Model file for the job. Use its own axes, mm. Round coordinates to 2 decimals unless told otherwise and drop trailing zeros. Loops run counter-clockwise (first coordinate to the right, second up) from the corner with the lowest first, then second, coordinate; pieces in that order, holes last. Notation, with made-up numbers: (51.5, 76.25) -> (58.5, 76.25) arc R13 ccw to (58.5, 96.25) -> close; hole circle Ø2 at (22.25, 82). An arc over 180 degrees is marked (long way). Use a Markdown table: item, result. Add a question column.
```python
from build123d import *

# Parameters (mm, degrees)
SKIZZE1_R                       = 2.25
AUFSATZ_LINEAR_AUSTRAGEN1_DEPTH = 20
SKIZZE2_R                       = 3
AUFSATZ_LINEAR_AUSTRAGEN2_DEPTH = 1
AUFSATZ_LINEAR_START            = 1
SKIZZE3_R                       = 3
AUFSATZ_LINEAR_AUSTRAGEN3_DEPTH = 1


with BuildPart() as part:
    # Skizze1 → Aufsatz-Linear austragen1 (new body)
    with BuildSketch(Plane.XY):
        with Locations((-14.9, 25)):
            Circle(SKIZZE1_R)
    extrude(amount=-AUFSATZ_LINEAR_AUSTRAGEN1_DEPTH)

    # Skizze2 → Aufsatz-Linear austragen2 (add)
    with BuildSketch(Plane.XY):
        with Locations((-14.9, 25)):
            Circle(SKIZZE2_R)
    extrude(amount=AUFSATZ_LINEAR_AUSTRAGEN2_DEPTH)

    # Skizze3 → Aufsatz-Linear austragen3 (add)
    with BuildSketch(Plane(origin=(0, 0, -20), x_dir=(-1, 0, 0), z_dir=(0, 0, -1)).offset(AUFSATZ_LINEAR_START)):
        with Locations(Location((14.9, 25, 0), (0, 0, 180))):
            Circle(SKIZZE3_R)
    extrude(amount=-AUFSATZ_LINEAR_AUSTRAGEN3_DEPTH)


solid = part.part
```
1) Cut at B-B on x = -14.9. Write the cut outline in (y, z), and give its area (3 significant figures).
2) Cut at C-C on z = -17.25. Write the cut outline in (x, y).
3) Pull direction Z, two halves, no side cores. Call faces 1 (the face through (-15, 25, -21)), 2 (the face through (-17.9, 25.1, 0.5)), 3 (the face through (-13.862, 23.004, -9.86)): +Z half, -Z half, draft (parallel to the pull), parting line (faces both ways), or undercut.
4) Wall check: probe 1 along Z at (x, y) = (-12.8, 26.4); probe 2 along Y at (x, z) = (-16.4, -19.5); probe 3 along X at (y, z) = (24.4, -15). Give the ranges that are in metal, low to high. Write a range as from..to.
5) Pin check, flat tips, straight feed: pin 1 Ø3 at (x, z) = (-14, -16.5) entering from -Y; pin 2 Ø3 at (y, z) = (24, -17.5) entering from +X. Stop position of each tip, or through.
6) Cut at A-A on y = 25. Write the cut outline in (x, z), and give its area (3 significant figures).
Established:
| question | item | result |
|---|---|---|
| 1 | outline | (22, -21) -> (28, -21) -> (28, -20) -> (27.25, -20) -> (27.25, 0) -> (28, 0) -> (28, 1) -> (22, 1) -> (22, 0) -> (22.75, 0) -> (22.75, -20) -> (22, -20) -> close |
| 1 | area | 102 mm^2 |
| 2 | outline | circle Ø4.5 at (-14.9, 25) |
| 3 | face 1 | -Z half |
| 3 | face 2 | draft |
| 3 | face 3 | undercut |
| 4 | probe 1 | z = -21..-20, 0..1 |
| 4 | probe 2 | y = 23.32..26.68 |
| 4 | probe 3 | x = -17.07..-12.73 |
| 5 | pin 1 | stops at y = 22.75 |
| 5 | pin 2 | stops at x = -12.65 |
| 6 | outline | (-17.9, -21) -> (-11.9, -21) -> (-11.9, -20) -> (-12.65, -20) -> (-12.65, 0) -> (-11.9, 0) -> (-11.9, 1) -> (-17.9, 1) -> (-17.9, 0) -> (-17.15, 0) -> (-17.15, -20) -> (-17.9, -20) -> close |
| 6 | area | 102 mm^2 |
